Part model, mm, in its own coordinate system. Give positions to 0.01 mm unless a question says otherwise; leave off trailing zeros. Loops run counter-clockwise (first coordinate to the right, second up) from the corner with the lowest first, then second, coordinate; pieces in that order, holes last. Notation, with made-up numbers: M -12,9 L 21,9 A4 cw 21,14 Z; hole C 42.5,22.5 d1. An arc over 180 degrees is marked long. Answer in a Markdown table with one row per item.
from build123d import *

# Parameters (mm, degrees)
SZKIC1_W                    = 596
SZKIC1_H                    = 496
DODANIE_WYCI_GNI_CIE1_DEPTH = 36
SZKIC2_R                    = 21
WYTNIJ_WYCI_GNI_CIE1_DEPTH  = 36
SZKIC3_R                    = 21
WYTNIJ_WYCI_GNI_CIE2_DEPTH  = 36
SZKIC4_R                    = 21
WYTNIJ_WYCI_GNI_CIE3_DEPTH  = 36
SZKIC5_R                    = 21
WYTNIJ_WYCI_GNI_CIE4_DEPTH  = 36
SZKIC6_W                    = 15
SZKIC6_H                    = 9
SZKIC7_W                    = 15
SZKIC7_H                    = 9
SZKIC8_W                    = 15
SZKIC8_H                    = 9
SZKIC9_W                    = 15
SZKIC9_H                    = 9
SZKIC10_W                   = 21
SZKIC10_H                   = 13
SZKIC11_W                   = 21
SZKIC11_H                   = 13
SZKIC12_W                   = 21
SZKIC12_H                   = 13
SZKIC13_W                   = 21
SZKIC13_H                   = 13


with BuildPart() as part:
    # Szkic1 → Dodanie-wyci_gni_cie1 (new body)
    with BuildSketch(Plane.XY):
        Rectangle(SZKIC1_W, SZKIC1_H)
    extrude(amount=DODANIE_WYCI_GNI_CIE1_DEPTH)

    # Szkic2 → Wytnij-wyci_gni_cie1 (cut)
    with BuildSketch(Plane.XY.offset(36)):
        with Locations((262, 162)):
            Circle(SZKIC2_R)
    extrude(amount=-WYTNIJ_WYCI_GNI_CIE1_DEPTH, mode=Mode.SUBTRACT)

    # Szkic3 → Wytnij-wyci_gni_cie2 (cut)
    with BuildSketch(Plane.XY.offset(36)):
        with Locations((262, -162)):
            Circle(SZKIC3_R)
    extrude(amount=-WYTNIJ_WYCI_GNI_CIE2_DEPTH, mode=Mode.SUBTRACT)

    # Szkic4 → Wytnij-wyci_gni_cie3 (cut)
    with BuildSketch(Plane.XY.offset(36)):
        with Locations((-262, -162)):
            Circle(SZKIC4_R)
    extrude(amount=-WYTNIJ_WYCI_GNI_CIE3_DEPTH, mode=Mode.SUBTRACT)

    # Szkic5 → Wytnij-wyci_gni_cie4 (cut)
    with BuildSketch(Plane.XY.offset(36)):
        with Locations((-262, 162)):
            Circle(SZKIC5_R)
    extrude(amount=-WYTNIJ_WYCI_GNI_CIE4_DEPTH, mode=Mode.SUBTRACT)

    # Szkic6 → Wyci_cie-obr_t1 (revolve, cut)
    with BuildSketch(Plane(origin=(215, 0, 0), x_dir=(0, 0, -1), z_dir=(1, 0, 0)), mode=Mode.PRIVATE) as wyci_cie_obr_t1_sk:
        with Locations((-7.5, 166.5)):
            Rectangle(SZKIC6_W, SZKIC6_H)
    revolve(wyci_cie_obr_t1_sk.sketch.rotate(Axis((215, 162, 0), (0, 0, 1)), 270), axis=Axis((215, 162, 0), (0, 0, 1)), mode=Mode.SUBTRACT)

    # Szkic7 → Wyci_cie-obr_t2 (revolve, cut)
    with BuildSketch(Plane(origin=(215, 0, 0), x_dir=(0, 0, -1), z_dir=(1, 0, 0)), mode=Mode.PRIVATE) as wyci_cie_obr_t2_sk:
        with Locations((-7.5, -166.5)):
            Rectangle(SZKIC7_W, SZKIC7_H)
    revolve(wyci_cie_obr_t2_sk.sketch.rotate(Axis((215, -162, 15), (0, 0, -1)), 90), axis=Axis((215, -162, 15), (0, 0, -1)), mode=Mode.SUBTRACT)

    # Szkic8 → Wyci_cie-obr_t3 (revolve, cut)
    with BuildSketch(Plane(origin=(-215, 0, 0), x_dir=(0, 0, -1), z_dir=(1, 0, 0)), mode=Mode.PRIVATE) as wyci_cie_obr_t3_sk:
        with Locations((-7.5, 166.5)):
            Rectangle(SZKIC8_W, SZKIC8_H)
    revolve(wyci_cie_obr_t3_sk.sketch.rotate(Axis((-215, 162, 0), (0, 0, 1)), 270), axis=Axis((-215, 162, 0), (0, 0, 1)), mode=Mode.SUBTRACT)

    # Szkic9 → Wyci_cie-obr_t4 (revolve, cut)
    with BuildSketch(Plane(origin=(-215, 0, 0), x_dir=(0, 0, -1), z_dir=(1, 0, 0)), mode=Mode.PRIVATE) as wyci_cie_obr_t4_sk:
        with Locations((-7.5, -166.5)):
            Rectangle(SZKIC9_W, SZKIC9_H)
    revolve(wyci_cie_obr_t4_sk.sketch.rotate(Axis((-215, -162, 15), (0, 0, -1)), 90), axis=Axis((-215, -162, 15), (0, 0, -1)), mode=Mode.SUBTRACT)

    # Szkic10 → Wyci_cie-obr_t5 (revolve, cut)
    with BuildSketch(Plane(origin=(215, 0, 0), x_dir=(0, 0, -1), z_dir=(1, 0, 0)), mode=Mode.PRIVATE) as wyci_cie_obr_t5_sk:
        with Locations((-25.5, 168.5)):
            Rectangle(SZKIC10_W, SZKIC10_H)
    revolve(wyci_cie_obr_t5_sk.sketch.rotate(Axis((215, 162, 15), (0, 0, 1)), 270), axis=Axis((215, 162, 15), (0, 0, 1)), mode=Mode.SUBTRACT)

    # Szkic11 → Wyci_cie-obr_t6 (revolve, cut)
    with BuildSketch(Plane(origin=(215, 0, 0), x_dir=(0, 0, -1), z_dir=(1, 0, 0)), mode=Mode.PRIVATE) as wyci_cie_obr_t6_sk:
        with Locations((-25.5, -168.5)):
            Rectangle(SZKIC11_W, SZKIC11_H)
    revolve(wyci_cie_obr_t6_sk.sketch.rotate(Axis((215, -162, 36), (0, 0, -1)), 90), axis=Axis((215, -162, 36), (0, 0, -1)), mode=Mode.SUBTRACT)

    # Szkic12 → Wyci_cie-obr_t7 (revolve, cut)
    with BuildSketch(Plane(origin=(-215, 0, 0), x_dir=(0, 0, -1), z_dir=(1, 0, 0)), mode=Mode.PRIVATE) as wyci_cie_obr_t7_sk:
        with Locations((-25.5, -168.5)):
            Rectangle(SZKIC12_W, SZKIC12_H)
    revolve(wyci_cie_obr_t7_sk.sketch.rotate(Axis((-215, -162, 36), (0, 0, -1)), 90), axis=Axis((-215, -162, 36), (0, 0, -1)), mode=Mode.SUBTRACT)

    # Szkic13 → Wyci_cie-obr_t8 (revolve, cut)
    with BuildSketch(Plane(origin=(-215, 0, 0), x_dir=(0, 0, -1), z_dir=(1, 0, 0)), mode=Mode.PRIVATE) as wyci_cie_obr_t8_sk:
        with Locations((-25.5, 168.5)):
            Rectangle(SZKIC13_W, SZKIC13_H)
    revolve(wyci_cie_obr_t8_sk.sketch.rotate(Axis((-215, 162, 15), (0, 0, 1)), 270), axis=Axis((-215, 162, 15), (0, 0, 1)), mode=Mode.SUBTRACT)


solid = part.part
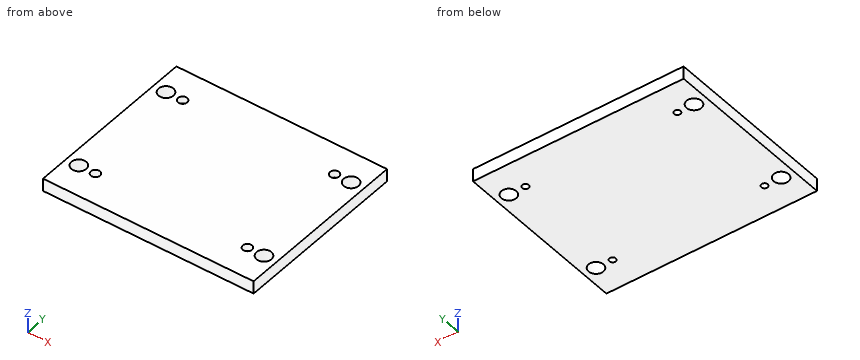
(1) Saw through at C-C (z = 22). Give the number of separate pieces and of enclosed holes in the cut face, plus the area to 3 significant figures.
Recorded:
| item | result |
|---|---|
| separate pieces | 1 |
| enclosed holes | 8 |
| area | 288,000 mm^2 |
(2) Pin check, flat tip, straight feed: pin 1 Ø21 at (x, y) = (-215, 162) entering from +Z. Stop position of the tip, or through.
Recorded:
| item | result |
|---|---|
| pin 1 | stops at z = 15 |
(3) Drill centre lines: line 1 along Y through (x, z) = (-262, 10); line 2 along Y through (x, z) = (215, 3). Where is each one in solid material? Low to high.
Recorded:
| item | result |
|---|---|
| line 1 | y = -248 to -183, -141 to 141, 183 to 248 |
| line 2 | y = -248 to -171, -153 to 153, 171 to 248 |
(4) Saw through at A-A (y = -162). Write the cut outline in (x, z).
Recorded:
| item | result |
|---|---|
| outline | M -298,0 L -283,0 L -283,36 L -298,36 Z; M -241,0 L -224,0 L -224,15 L -228,15 L -228,36 L -241,36 Z; M -206,0 L 206,0 L 206,15 L 202,15 L 202,36 L -202,36 L -202,15 L -206,15 Z; M 224,0 L 241,0 L 241,36 L 228,36 L 228,15 L 224,15 Z; M 283,0 L 298,0 L 298,36 L 283,36 Z |
(5) Saw through at B-B (x = -262). Write the cut outline in (y, z).
Recorded:
| item | result |
|---|---|
| outline | M -248,0 L -183,0 L -183,36 L -248,36 Z; M -141,0 L 141,0 L 141,36 L -141,36 Z; M 183,0 L 248,0 L 248,36 L 183,36 Z |
(6) Saw through at D-D (x = 254). Write the cut outline in (y, z).
Recorded:
| item | result |
|---|---|
| outline | M -248,0 L -181.42,0 L -181.42,36 L -248,36 Z; M -142.58,0 L 142.58,0 L 142.58,36 L -142.58,36 Z; M 181.42,0 L 248,0 L 248,36 L 181.42,36 Z |
